Input: part model. Units: mm. Frame: model coordinates. A direction names the side the tool comes from. Round coordinates to 2 decimals unless told otherwise and drop trailing zeros. Loops run counter-clockwise (first coordinate to the right, second up) from the corner with the lowest first, then second, coordinate; pieces in that order, holes last.
(1) Cut plane A-A, the plane x = 0. Output: boundary loops of the cut face in (y, z), and give its area (3 significant figures).
(2) First-contact query: pin 1 Ø4 at (x, y) = (-7, 17.5) entering from -Z; pin 2 Ø2 at (x, y) = (44, 9) entering from -Z; pin 3 Ø2 at (y, z) = (27.5, 4.5) entering from +X; pin 4 Ø1 at (x, z) = (-53.5, -52) entering from -Y. Flat tips, straight axial feed; report the tip coordinate or a pass-through.
(3) Cut plane B-B, the plane z = 0. Output: boundary loops of the cut face in (x, y).
(4) Cut plane C-C, the plane y = 10. Output: boundary loops of the cut face in (x, z), and give its area (3 significant figures).
(5) Access query for faces 1 (the face through (14, 45, -14)), 2 (the face through (-19.52, 43.77, -62)). Directions: +Z, -Z, +X, -X, +Y, -Y. A direction counts if a zero-diameter tool reaches every point of the face in a straight line with its end or side. Return the directions, or none.
(6) Line query: line 1 (X direction, y = 14, z = 0); line 2 (Z direction, x = -1, y = 36.5); line 3 (Z direction, x = 10, y = 27). Output: solid intervals per line, ascending.
(7) Draft query along Z for faces 3 (the face through (64.5, 40, -21.3)), 4 (the face through (64.32, 17.74, -33.45)), 5 (the face through (17.084, 22.185, 3.794)). Return one class per face: released by +Z, released by -Z, zero draft, split by the parting line, or undercut.
from build123d import *


with BuildPart() as part:
    # 草图1 → 旋转1 (revolve)
    with BuildSketch(Plane(origin=(0, 0, 0), x_dir=(0, 0, -1), z_dir=(1, 0, 0)), mode=Mode.PRIVATE) as revolve_1_sk:
        with BuildLine():
            Line((-17.5, 45), (-17.5, 0))
            Line((-17.5, 0), (-72.5, 0))
            Line((-72.5, 0), (-72.5, 35))
            Line((-72.5, 35), (-72.9, 35))
            Line((-72.9, 35), (-72.9, 40))
            Line((-72.9, 40), (-67.5, 40))
            ThreePointArc((-67.5, 40), (-65.732233047, 40.732233047), (-65, 42.5))
            Line((-65, 42.5), (-65, 45))
            Line((-65, 45), (-17.5, 45))
        make_face()
    revolve(revolve_1_sk.sketch.rotate(Axis((0, 0, 0), (0, 1, 0)), 180), axis=Axis((0, 0, 0), (0, 1, 0)))


solid = part.part
Reported:
1. outline: (0, -72.5) - (35, -72.5) - (35, -72.9) - (40, -72.9) - (40, -67.5) arc R2.5 cw to (42.5, -65) - (45, -65) - (45, -17.5) - (0, -17.5) - close; (0, 17.5) - (45, 17.5) - (45, 65) - (42.5, 65) arc R2.5 cw to (40, 67.5) - (40, 72.9) - (35, 72.9) - (35, 72.5) - (0, 72.5) - close
1. area: 4,880 mm2
2. pin 1: stops at z = -72.33
2. pin 2: stops at z = -58.37
2. pin 3: stops at x = 72.42
2. pin 4: passes through
3. outline: (-72.9, 35) - (-72.5, 35) - (-72.5, 0) - (-17.5, 0) - (-17.5, 45) - (-65, 45) - (-65, 42.5) arc R2.5 cw to (-67.5, 40) - (-72.9, 40) - close; (17.5, 0) - (72.5, 0) - (72.5, 35) - (72.9, 35) - (72.9, 40) - (67.5, 40) arc R2.5 cw to (65, 42.5) - (65, 45) - (17.5, 45) - close
4. outline: circle Ø145 at (0, 0); hole circle Ø35 at (0, 0)
4. area: 15,600 mm2
5. face 1: +Z, -Z, +X, -X, +Y
5. face 2: +Y
6. line 1: x = -72.5 to -17.5, 17.5 to 72.5
6. line 2: z = -72.89 to -17.47, 17.47 to 72.89
6. line 3: z = -71.81 to -14.36, 14.36 to 71.81
7. face 3: zero draft
7. face 4: split by the parting line
7. face 5: undercut
